Here's the drawing with two shaded views (mm, measured from the low corner). I have some questions. A direction names the side the tool comes from. Coordinates: 2 decimals unless noted, no trailing zeros. Write each loop counter-clockwise with the first axis right and the second up, starting at its lowest first coordinate (ties: lowest second). Pieces come first, ordered by that corner, then holes.
Item 1: For P1, Ø2, axis at x = 425.5, z = 781.5, coming from the -Y side, with a flat end and sliding along its axis, tell me the tip position at first contact or that it passes through.
Item 2: I want a section at C-C on x = 655. Please give me the cut outline in (y, z), then the cut area to 3 significant figures.
Item 3: I want a section at A-A on z = 561.5. Please give me the cut outline in (x, y).
Item 4: I want a section at B-B on y = 180.5. Please give me the cut outline in (x, z).
Item 5: If I drill on probe 1 along X at (y, z) = (54, 497.5); probe 2 along Z at (x, y) = (1227.5, 142.5); probe 3 along Y at (x, z) = (1908, 771), over which ranges is the centre line in solid material (lowest first)?
Item 6: Thinking about a two-plate mould opening in X: for the marked faces 3, 4 and 5, which applies, +X half, -X half, draft (parallel to the pull), parting line (faces both ways), or undercut?
Item 7: Which directions (+Z, -Z, +X, -X, +Y, -Y) give clear straight access to the entire face, cutting with the end or side of a thin tool? Please do the marked faces 1 and 2.
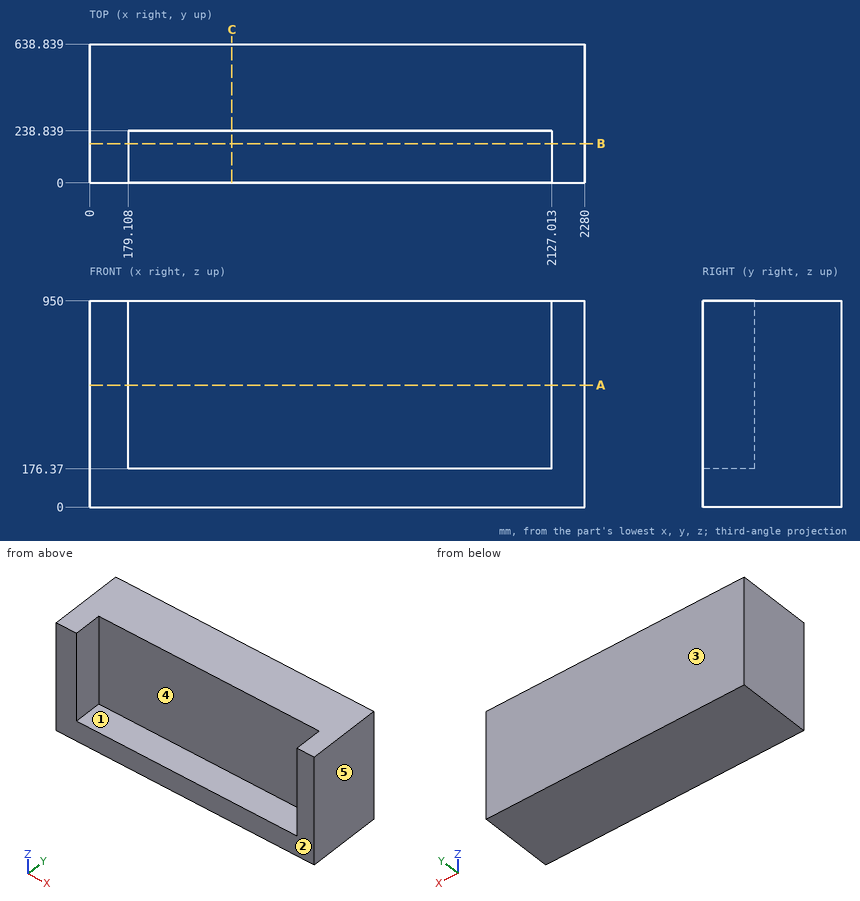
Response values:
1. P1: stops at y = 238.84
2. outline: (0, 0) - (638.84, 0) - (638.84, 950) - (238.84, 950) - (238.84, 176.37) - (0, 176.37) - close
2. area: 422,000 mm2
3. outline: (0, 0) - (179.11, 0) - (179.11, 238.84) - (2127.01, 238.84) - (2127.01, 0) - (2280, 0) - (2280, 638.84) - (0, 638.84) - close
4. outline: (0, 0) - (2280, 0) - (2280, 950) - (2127.01, 950) - (2127.01, 176.37) - (179.11, 176.37) - (179.11, 950) - (0, 950) - close
5. probe 1: x = 0 to 179.11, 2127.01 to 2280
5. probe 2: z = 0 to 176.37
5. probe 3: y = 238.84 to 638.84
6. face 3: draft
6. face 4: undercut
6. face 5: +X half
7. face 1: +Z, -Y
7. face 2: +Z, -Z, +X, -X, -Y
